Autodesk Inventor part; units mm, degrees
ref_plane "YZ Plane" through (0, 0, 0) normal (1, 0, 0) x (0, 1, 0)
ref_plane "XZ Plane" through (0, 0, 0) normal (0, 1, 0) x (-1, 0, 0)
ref_plane "XY Plane" through (0, 0, 0) normal (0, 0, 1) x (1, 0, 0)
sketch "Sketch1" plane through (0, 0, 0) normal (0, 0, 1) x (1, 0, 0)
  line L0 (0, 11.2) -> (0, -11.2)
  line L1 (-11.2, 0) -> (11.2, 0)
  line L2 (-8, 8) -> (8, 8)
  line L3 (8, 8) -> (8, -8)
  line L4 (8, -8) -> (-8, -8)
  line L5 (-8, -8) -> (-8, 8)
  dimension "d0" = 16
  dimension "d1" = 16
extrude "BLOK" add sketch "Sketch1" along normal mid plane 9
sketch "Sketch3" plane through (-8, -8, 4.5) normal (-1, 0, 0) x (0, 0, 1)
  line L0 (0, 0) -> (-9, 0)
  line L1 (-9, 16) -> (0, 16)
  line L2 (-9, 0) -> (-9, 16)
  line L3 (-7, 15) -> (-2, 15)
  line L4 (-2, 15) -> (-2, 1)
  line L5 (-2, 1) -> (-7, 1)
  line L6 (-7, 1) -> (-7, 15)
  point P0 (-4.5, 8)
  dimension "d21" = 2
  dimension "d22" = 1
  dimension "d23" = 1
  dimension "d24" = 5
extrude "USBGAT" cut sketch "Sketch3" against normal blind 12
properties part number "USB_Cap"
Design review of the part built by this model. Coordinates are the model's own, in mm. A direction names the side the tool comes from. Coordinates: 2 decimals unless noted, no trailing zeros. Loops run counter-clockwise (first coordinate to the right, second up) from the corner with the lowest first, then second, coordinate; pieces in that order, holes last. Notation, with made-up numbers: (57.25, 70) - (91.25, 70) arc R26 ccw to (91.25, 103) - close; hole circle Ø5 at (-21.5, -21.75). An arc over 180 degrees is marked (long way). Use CSV: the item, a comma, the result in double quotes. Start each with the question number.
1) Tool access review of faces 1 (the flat face through (4, 0, 0)), 2 (the flat face through (-8, 0, -3)): name each direction out of +Z, -Z, +X, -X, +Y, -Y from which nothing blocks a thin tool from reaching the whole face with its end or side.
2) Consider section C-C on z = 0.25. Write out the cut boundary in (x, y).
3) Consider section A-A on y = 3.75. Write out the cut boundary in (x, z).
4) Consider section B-B on x = 1.75. Write out the cut boundary in (y, z), then the cut area to 3 significant figures.
5) Wall thickness on L1, parallel to Z at x = 1.5, y = -5; L2, parallel to Y at x = -4.5, z = 1.25; L3, parallel to X at y = 5, z = 1.25: over which ranges is each line inside the solid? List them lowest first. Write a range as from..to.
6) The part is to be moulded in two halves that separate along Y. For faces 3 (the flat face through (-2, -7, 0)), 4 (the flat face through (0, 0, -4.5)), 5 (the flat face through (0, -8, 0)), 6 (the flat face through (-2, 7, 0)), say which applies: +Y half, -Y half, draft (parallel to the pull), parting line (faces both ways), or undercut.
Geometry says:
1,face 1,"-X"
1,face 2,"+Z, -Z, -X, +Y, -Y"
2,outline,"(-8, -8) - (8, -8) - (8, 8) - (-8, 8) - (-8, 7) - (4, 7) - (4, -7) - (-8, -7) - close"
3,outline,"(-8, -4.5) - (8, -4.5) - (8, 4.5) - (-8, 4.5) - (-8, 2.5) - (4, 2.5) - (4, -2.5) - (-8, -2.5) - close"
4,outline,"(-8, -4.5) - (8, -4.5) - (8, 4.5) - (-8, 4.5) - close; hole (-7, -2.5) - (7, -2.5) - (7, 2.5) - (-7, 2.5) - close"
4,area,"74.0 mm^2"
5,L1,"-4.5..-2.5, 2.5..4.5"
5,L2,"-8..-7, 7..8"
5,L3,"4..8"
6,face 3,"undercut"
6,face 4,"draft"
6,face 5,"-Y half"
6,face 6,"undercut"
